Part model, mm, in its own coordinate system. A direction names the side the tool comes from. Coordinates: 2 decimals unless noted, no trailing zeros. Write each loop counter-clockwise with the first axis right and the second up, starting at its lowest first coordinate (ties: lowest second). Pieces come first, ordered by that corner, then holes. Notation, with made-up numbers: (-16, 36.25) - (6, 36.25) arc R22 ccw to (6, 65.25) - close; hole circle Ø7 at (7.25, 37.25). An arc over 180 degrees is marked (long way). Use a Markdown table: item, result.
```python
from build123d import *

# Parameters (mm, degrees)
F2_DEPTH = 25
F3_W     = 204.2875885963
F3_H     = 330.4814696312
F4_DEPTH = 25


with BuildPart() as f2:
    # F1 (on Top) → F2 (new body)
    with BuildSketch(Plane.XY):
        with BuildLine():
            Line((168.3422140292, 474.8379558081), (181.0361660289, 474.454610266))
            ThreePointArc((181.0361660289, 474.454610266), (174.8820955467, 481.0340797179), (168.3422140292, 474.8379558081))
        make_face()
        with BuildLine():
            Line((166.6445245232, 81.42426457), (181.0361660289, 474.454610266))
            Line((181.0361660289, 474.454610266), (168.3422140292, 474.8379558081))
            Line((168.3422140292, 474.8379558081), (-166.9943213011, 484.9648072356))
            Line((-166.9943213011, 484.9648072356), (-178.021518384, 183.8161801091))
            add(Edge.make_bspline(
                [(-178.021518384, 183.8161801091), (-126.121723234, 189.1373544028), (-5.2720297028, 157.9893070947), (124.2923755779, 80.293310388), (162.9702843725, 49.4019598786)],
                knots=[504.1665264406, 504.1665264406, 504.1665264406, 504.1665264406, 653.3978700476, 795.436226982, 795.436226982, 795.436226982, 795.436226982], degree=3))
            add(Edge.make_bspline(
                [(162.9702843725, 49.4019598786), (163.7914086642, 48.7461426667), (164.6014886785, 48.0934791624), (165.4002701181, 47.4441422338)],
                knots=[795.436226982, 795.436226982, 795.436226982, 795.436226982, 798.4516729787, 798.4516729787, 798.4516729787, 798.4516729787], degree=3))
            Line((165.4002701181, 47.4441422338), (166.6445245232, 81.42426457))
        make_face()
        with BuildLine():
            Line((163.474066231, -5.1597653413), (165.4002701181, 47.4441422338))
            add(Edge.make_bspline(
                [(162.9702843725, 49.4019598786), (163.7914086642, 48.7461426667), (164.6014886785, 48.0934791624), (165.4002701181, 47.4441422338)],
                knots=[795.436226982, 795.436226982, 795.436226982, 795.436226982, 798.4516729787, 798.4516729787, 798.4516729787, 798.4516729787], degree=3))
            Line((162.9702843725, 49.4019598786), (160.9759493271, -5.0625841432))
            add(Edge.make_bspline(
                [(163.474066231, -5.1597653413), (162.6521846932, -5.131062894), (161.8193790258, -5.0986033684), (160.9759493271, -5.0625841432)],
                knots=[958.9382746439, 958.9382746439, 958.9382746439, 958.9382746439, 961.7589781967, 961.7589781967, 961.7589781967, 961.7589781967], degree=3))
        make_face()
        with BuildLine():
            Line((160.9759493271, -5.0625841432), (162.9702843725, 49.4019598786))
            add(Edge.make_bspline(
                [(-178.021518384, 183.8161801091), (-126.121723234, 189.1373544028), (-5.2720297028, 157.9893070947), (124.2923755779, 80.293310388), (162.9702843725, 49.4019598786)],
                knots=[504.1665264406, 504.1665264406, 504.1665264406, 504.1665264406, 653.3978700476, 795.436226982, 795.436226982, 795.436226982, 795.436226982], degree=3))
            Line((-178.021518384, 183.8161801091), (-181.3042814193, 94.1651496755))
            Line((-181.3042814193, 94.1651496755), (-88.1747823589, -19.1265900522))
            add(Edge.make_bspline(
                [(160.9759493271, -5.0625841432), (121.4037743321, -3.3726281412), (19.2880670567, 12.0779258477), (-62.8138782039, -5.4855367148), (-88.1747823589, -19.1265900522)],
                knots=[961.7589781967, 961.7589781967, 961.7589781967, 961.7589781967, 1094.1012170077, 1176.4100957539, 1176.4100957539, 1176.4100957539, 1176.4100957539], degree=3))
        make_face()
        with BuildLine():
            Line((159.4487037703, -115.0909082779), (163.474066231, -5.1597653413))
            add(Edge.make_bspline(
                [(163.474066231, -5.1597653413), (162.6521846932, -5.131062894), (161.8193790258, -5.0986033684), (160.9759493271, -5.0625841432)],
                knots=[958.9382746439, 958.9382746439, 958.9382746439, 958.9382746439, 961.7589781967, 961.7589781967, 961.7589781967, 961.7589781967], degree=3))
            add(Edge.make_bspline(
                [(160.9759493271, -5.0625841432), (121.4037743321, -3.3726281412), (19.2880670567, 12.0779258477), (-62.8138782039, -5.4855367148), (-88.1747823589, -19.1265900522)],
                knots=[961.7589781967, 961.7589781967, 961.7589781967, 961.7589781967, 1094.1012170077, 1176.4100957539, 1176.4100957539, 1176.4100957539, 1176.4100957539], degree=3))
            Line((-88.1747823589, -19.1265900522), (152.2528830175, -311.6060811259))
            Line((152.2528830175, -311.6060811259), (155.8507933939, -213.3484947019))
            Line((155.8507933939, -213.3484947019), (159.4487037703, -115.0909082779))
        make_face()
    extrude(amount=F2_DEPTH)

    # F3 (on face) → F4 (join)
    with BuildSketch(Plane.XZ):
        with Locations((-3.8982927799, 14.3264830112)):
            Rectangle(F3_W, F3_H)
    extrude(amount=F4_DEPTH)


solid = f2.part
```
Item 1: Band-saw the part on C-C, the plane y = -162.5. Give the cut face in (x, z).
From the geometry:
| item | result |
|---|---|
| outline | (29.68, 0) - (157.71, 0) - (157.71, 25) - (29.68, 25) - close |
Item 2: Band-saw the part on B-B, the plane z = -125. Give the cut face in (x, y).
From the geometry:
| item | result |
|---|---|
| outline | (-106.04, -25) - (98.25, -25) - (98.25, 0) - (-106.04, 0) - close |
Item 3: Which spindle directions (+Z, -Z, +X, -X, +Y, -Y) get a long thin tool onto all of the face, cutting with end or side? Do faces 1 (the face through (98.246, -12, 101)), 2 (the face through (166.443, 75.922, 12.325)). Say none if no direction does.
From the geometry:
| item | result |
|---|---|
| face 1 | +Z, +X, +Y, -Y |
| face 2 | +Z, -Z, +X, -Y |
Item 4: Drop flat-ended pins along their axis: P1, Ø7.5, axis at y = -16, z = 103.5, coming from the +X side; P2, Ø6, axis at x = -134.5, y = 275.5, coming from the +Z side; P3, Ø1.5, axis at x = 135.5, y = 254.5, coming from the -Z side; P4, Ø5, axis at x = -110, y = -27.5, coming from the -Z side. Give the stop position or say it passes through.
From the geometry:
| item | result |
|---|---|
| P1 | x = 98.25 |
| P2 | z = 25 |
| P3 | z = 0 |
| P4 | through |
Item 5: Two-plate mould, pull along X, no slides. Class faces 3 (the face through (98.246, -12, -77)), 4 (the face through (-174.05, 292.3, 12.32)), 5 (the face through (-3, 181, 0)): pulls with the +X half, pulls with the -X half, needs draft (parallel to the pull), parting line crosses it, or undercut.
From the geometry:
| item | result |
|---|---|
| face 3 | pulls with the +X half |
| face 4 | pulls with the -X half |
| face 5 | needs draft |
Item 6: Drill centre lines: probe 1 along Z at (x, y) = (-143, 443); probe 2 along Y at (x, z) = (-51.5, -56); probe 3 along X at (y, z) = (-99, 23). Where is each one in solid material? Low to high.
From the geometry:
| item | result |
|---|---|
| probe 1 | 0 to 25 |
| probe 2 | -25 to 0 |
| probe 3 | -22.52 to 160.04 |
Item 7: Band-saw the part on D-D, the plane x = -34.5. Give the cut face in (y, z), then the cut area to 3 significant figures.
From the geometry:
| item | result |
|---|---|
| outline | (-84.42, 0) - (-25, 0) - (-25, -150.91) - (0, -150.91) - (0, 0) - (480.96, 0) - (480.96, 25) - (0, 25) - (0, 179.57) - (-25, 179.57) - (-25, 25) - (-84.42, 25) - close |
| area | 21,800 mm^2 |
Item 8: Band-saw the part on A-A, the plane x = 61.5. Give the cut face in (y, z), then the cut area to 3 significant figures.
From the geometry:
| item | result |
|---|---|
| outline | (-201.21, 0) - (-25, 0) - (-25, -150.91) - (0, -150.91) - (0, 0) - (478.06, 0) - (478.06, 25) - (0, 25) - (0, 179.57) - (-25, 179.57) - (-25, 25) - (-201.21, 25) - close |
| area | 24,600 mm^2 |
